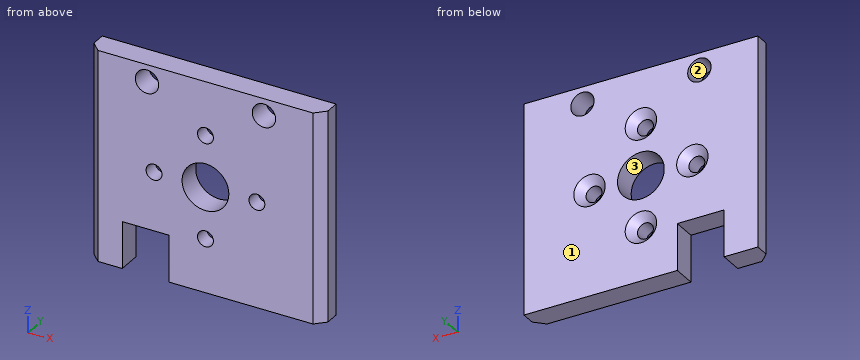
```python
from build123d import *

# Parameters (mm, degrees)
F0_R           = 1.5
F0_R_2         = 2.5
F0_R_3         = 5
F1_DEPTH       = 5
F2_D           = 3.4
F2_CSINK_D     = 6.72
F2_CSINK_ANGLE = 90
F3_SIZE        = 2


with BuildPart() as f1:
    # F0 (on Front) → F1 (new body)
    with BuildSketch(Plane.XZ):
        Polygon((25, -22.5), (25, 22.5), (-25, 22.5), (-25, -22.5), (-17.784204334, -22.5), (-17.784204334, -12.5), (-7.784204334, -12.5), (-7.784204334, -22.5), align=None)
        with Locations((0, -11)):
            Circle(F0_R, mode=Mode.SUBTRACT)
        with Locations((-11, 0)):
            Circle(F0_R, mode=Mode.SUBTRACT)
        with Locations((-12.5, 18.8740361482)):
            Circle(F0_R_2, mode=Mode.SUBTRACT)
        Circle(F0_R_3, mode=Mode.SUBTRACT)
        with Locations((11, 0)):
            Circle(F0_R, mode=Mode.SUBTRACT)
        with Locations((0, 11)):
            Circle(F0_R, mode=Mode.SUBTRACT)
        with Locations((12.5, 18.8740361482)):
            Circle(F0_R_2, mode=Mode.SUBTRACT)
    extrude(amount=F1_DEPTH)

    # F2 (through all)
    with Locations(Plane(origin=(0, 0, 0), x_dir=(1, 0, 0), z_dir=(0, 1, 0))):
        with Locations((-11, 0), (11, 0), (0, -11), (0, 11)):
            CounterSinkHole(F2_D / 2, F2_CSINK_D / 2, counter_sink_angle=F2_CSINK_ANGLE)

    # F3
    f3_edges = [f1.edges().sort_by_distance(p)[0] for p in [
        (25, -5, 0),
        (-25, -5, 0),
    ]]
    chamfer(f3_edges, length=F3_SIZE)


solid = f1.part
```
CAD build for the part. Positions are in the model's coordinates, mm. Face numbers are marked on the shaded views. Round coordinates to 2 decimals unless told otherwise and drop trailing zeros. Order: outer loops, then holes, each group sorted by start corner. A loop starts at its lowest first (then second) coordinate and runs counter-clockwise, first axis right, second up. Notation, with made-up numbers: (49.25, -10.5) - (66.25, -10.5) arc R16 ccw to (66.25, 7.5) - close; hole circle Ø6 at (-14, 69.25). An arc over 180 degrees is marked (long way). Use CSV: the item, a comma, the result in double quotes. Start each with the question number.
1) Pin check, flat tip, straight feed: pin 1 Ø4 at (x, z) = (11, 0) entering from +Y. Stop position of the tip, or through.
2) Saw through at B-B (x = 0). List the corners of the cut face in (y, z).
3) Two-plate mould, pull along Z, no slides. Class the marked faces 1, 2 and 3: pulls with the +Z half, pulls with the -Z half, needs draft (parallel to the pull), parting line crosses it, or undercut.
4) Saw through at A-A (z = -17). List the corners of the cut face in (x, y), and give its area (3 significant figures).
5) Saw through at D-D (y = -3.55). List the corners of the cut face in (x, z), and give its area (3 significant figures).
6) Saw through at C-C (z = 18). List the corners of the cut face in (x, y).
7) Wall check: L1, parallel to Z at x = 0, y = -2.5; L2, parallel to Z at x = 11.5, y = -2.4; L3, parallel to X at y = -2.45, z = -11. Give the ranges that are in metal, low to high. Write a range as [from, to].
Values follow:
1,pin 1,"stops at y = -1.36"
2,outline,"(-5, -22.5) - (0, -22.5) - (0, -14.36) - (-1.66, -12.7) - (-5, -12.7) - close; (-5, -9.3) - (-1.66, -9.3) - (0, -7.64) - (0, -5) - (-5, -5) - close; (-5, 5) - (0, 5) - (0, 7.64) - (-1.66, 9.3) - (-5, 9.3) - close; (-5, 12.7) - (-1.66, 12.7) - (0, 14.36) - (0, 22.5) - (-5, 22.5) - close"
3,face 1,"needs draft"
3,face 2,"undercut"
3,face 3,"undercut"
4,outline,"(-25, -3) - (-23, -5) - (-17.78, -5) - (-17.78, 0) - (-25, 0) - close; (-7.78, -5) - (23, -5) - (25, -3) - (25, 0) - (-7.78, 0) - close"
4,area,"196 mm2"
5,outline,"(-24.45, -22.5) - (-17.78, -22.5) - (-17.78, -12.5) - (-7.78, -12.5) - (-7.78, -22.5) - (24.45, -22.5) - (24.45, 22.5) - (-24.45, 22.5) - close; hole circle Ø5 at (-12.5, 18.87); hole circle Ø3.4 at (-11, 0); hole circle Ø10 at (0, 0); hole circle Ø3.4 at (0, -11); hole circle Ø3.4 at (0, 11); hole circle Ø3.4 at (11, 0); hole circle Ø5 at (12.5, 18.87)"
5,area,"1,950 mm2"
6,outline,"(-25, -3) - (-23, -5) - (-14.84, -5) - (-14.84, 0) - (-25, 0) - close; (-10.16, -5) - (10.16, -5) - (10.16, 0) - (-10.16, 0) - close; (14.84, -5) - (23, -5) - (25, -3) - (25, 0) - (14.84, 0) - close"
7,L1,"z = [-22.5, -12.7], [-9.3, -5], [5, 9.3], [12.7, 22.5]"
7,L2,"z = [-22.5, -1.62], [1.62, 16.58], [21.17, 22.5]"
7,L3,"x = [-25, -1.7], [1.7, 25]"
